Drawing for the job (mm, zero at the part's lowest x, y, z). Coordinates: 2 decimals unless noted, no trailing zeros. Write each loop counter-clockwise with the first axis right and the second up, starting at its lowest first coordinate (ties: lowest second). Pieces come first, ordered by that corner, then holes. Notation, with made-up numbers: (56.25, 53.25) - (96.25, 53.25) arc R38 ccw to (96.25, 92.25) - close; hole circle Ø1 at (20.5, 14). An arc over 180 degrees is marked (long way). Write each question's results on one line, items separated by ' | '.
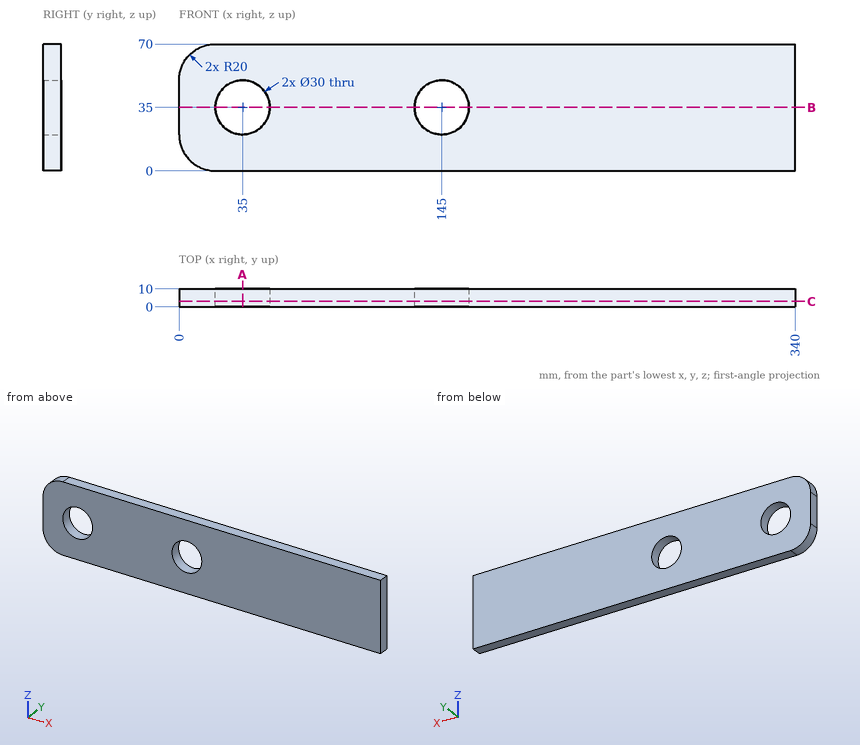
(1) Wall check: line 1 (X direction, y = 5.25, z = 35); line 2 (Z direction, x = 145, y = 6.5); line 3 (X direction, y = 1.75, z = 47). Give the ranges that are in metal, low to high. Write a range as from..to.
Return value:
line 1: x = 0..20, 50..130, 160..340 | line 2: z = 0..20, 50..70 | line 3: x = 0..26, 44..136, 154..340
(2) Saw through at A-A on x = 35. Write the cut outline in (y, z).
Return value:
outline: (0, 0) - (10, 0) - (10, 20) - (0, 20) - close; (0, 50) - (10, 50) - (10, 70) - (0, 70) - close
(3) Saw through at B-B on z = 35. Write the cut outline in (x, y), then the cut area to 3 significant figures.
Return value:
outline: (0, 0) - (20, 0) - (20, 10) - (0, 10) - close; (50, 0) - (130, 0) - (130, 10) - (50, 10) - close; (160, 0) - (340, 0) - (340, 10) - (160, 10) - close | area: 2,800 mm^2
(4) Saw through at C-C on y = 3. Write the cut outline in (x, z), then the cut area to 3 significant figures.
Return value:
outline: (0, 20) arc R20 ccw to (20, 0) - (340, 0) - (340, 70) - (20, 70) arc R20 ccw to (0, 50) - close; hole circle Ø30 at (35, 35); hole circle Ø30 at (145, 35) | area: 22,200 mm^2
